Autodesk Inventor part; units mm, degrees
ref_plane "YZ Plane" through (0, 0, 0) normal (1, 0, 0) x (0, 1, 0)
ref_plane "XZ Plane" through (0, 0, 0) normal (0, 1, 0) x (-1, 0, 0)
ref_plane "XY Plane" through (0, 0, 0) normal (0, 0, 1) x (1, 0, 0)
sketch "Sketch1" plane through (0, 0, 0) normal (0, 0, 1) x (1, 0, 0)
  line L0 (-30, 0) -> (0, 0)
  line L1 (100, 0) -> (0, 0)
  line L2 (100, 0) -> (100, -35)
  line L3 (100, -35) -> (5, -35)
  arc A0 (-30, 0) -> (5, -35) centre (5, 0) ccw
  dimension "d0" = 30
  dimension "d26" = 130
  dimension "d27" = 35
  dimension "d28" = 35
extrude "Extrusion1" add sketch "Sketch1" against normal blind 50
sketch "Sketch2" plane through (-30, 0, 0) normal (0, 1, 0) x (1, 0, 0)
  circle A0 centre (110, 25) radius 12.5
  circle A1 centre (110, 25) radius 35
  line L0 (0, 0) -> (0, 50)
  line L1 (0, 25) -> (130, 25)
  line L2 (130, 0) -> (130, 50)
  point P0 (30, 0)
  dimension "d6" = 25
  dimension "d7" = 70
  dimension "d8" = 110
extrude "Extrusion4" add sketch "Sketch2" against normal up to surface (35 mm away) contours L1 A0 | A1 | A0 L1
sketch "Sketch4" plane through (-30, 0, 0) normal (0, 1, 0) x (1, 0, 0)
  line L0 (85.5051, 0) -> (0, 0)
  line L1 (19, 0) -> (19, 9)
  line L2 (19, 9) -> (12, 9)
  line L3 (12, 9) -> (12, 12)
  line L4 (12, 12) -> (19, 12)
  line L5 (19, 12) -> (19, 27)
  line L6 (19, 27) -> (9, 27)
  line L7 (9, 27) -> (9, 47)
  line L8 (9, 47) -> (76, 47)
  line L9 (76, 47) -> (76, 0)
  line L10 (71, 0) -> (71, 42)
  line L11 (71, 42) -> (19, 42)
  line L12 (19, 42) -> (19, 40)
  line L13 (19, 40) -> (59, 40)
  line L14 (59, 40) -> (59, 12)
  line L15 (59, 12) -> (66, 12)
  line L16 (66, 12) -> (66, 9)
  line L17 (66, 9) -> (59, 9)
  line L18 (59, 9) -> (59, 0)
  point P0 (30, 0)
  point P1 (12, 10.5)
  point P2 (66, 10.5)
  dimension "d31" = 54
  dimension "d32" = 36
  dimension "d33" = 7
  dimension "d34" = 7
  dimension "d35" = 40
  dimension "d36" = 2
  dimension "d37" = 3
  dimension "d38" = 9
  dimension "d39" = 15
  dimension "d40" = 10
  dimension "d41" = 20
  dimension "d42" = 5
  dimension "d43" = 67
extrude "Extrusion5" cut sketch "Sketch4" against normal blind 10 contours L0 L10 L11 L12 L13 L14 L15 L16 L17 L18 L1 L2 L3 L4 L5 L6 L7 L8 L9
sketch "Sketch5" plane through (-30, 0, 0) normal (0, 1, 0) x (1, 0, 0)
  arc A0 (85.5051, 0) -> (85.5051, 50) centre (110, 25) ccw
  circle A1 centre (110, 25) radius 35
  circle A2 centre (110, 25) radius 12.5
  point P0 (30, 0)
  point P1 (85.5051, 50)
  point P2 (85.5051, 0)
  dimension "d46" = 25
extrude "Extrusion6" cut sketch "Sketch5" against normal blind 22.5 contours A1 A0 | A2
sketch "Sketch6" plane through (-30, -22.5, 0) normal (0, 1, 0) x (1, 0, 0)
  arc A0 (85.5051, 0) -> (85.5051, 50) centre (110, 25) ccw
  arc A1 (85.5051, 50) -> (85.5051, 0) centre (110, 25) ccw
  circle A2 centre (110, 25) radius 12.5
  point P0 (30, 0)
  dimension "d49" = 25
extrude "Extrusion7" cut sketch "Sketch6" against normal blind 5 contours A2
properties part number "wirst 2 left"
Part model, mm, in its own coordinate system. A direction names the side the tool comes from. Give positions to 0.01 mm unless a question says otherwise; leave off trailing zeros. Order: outer loops, then holes, each group sorted by start corner. A loop starts at its lowest first (then second) coordinate and runs counter-clockwise, first axis right, second up. Notation, with made-up numbers: (-23, 39.5) - (21, 39.5) arc R9 cw to (21, 56.5) - close; hole circle Ø7 at (41.25, 72.5). An arc over 180 degrees is marked (long way). Use a Markdown table: item, result.
1) Flat gauge pins, fed straight in: P1, Ø8, axis at x = 72.5, z = -2, coming from the +Y side; P2, Ø8, axis at y = -11.5, z = -8, coming from the +X side; P3, Ø5, axis at y = -6.5, z = -15, coming from the +X side. Where does each tip first touch, or does it go through?
Checked values:
| item | result |
|---|---|
| P1 | y = -22.5 |
| P2 | x = 52 |
| P3 | x = 47.31 |
2) Saw through at C-C on y = -3. List the corners of the cut face in (x, z).
Checked values:
| item | result |
|---|---|
| outline | (-29.87, -50) - (55.51, -50) arc R35 cw to (46, -33.31) - (46, -47) - (-21, -47) - (-21, -27) - (-11, -27) - (-11, -12) - (-18, -12) - (-18, -9) - (-11, -9) - (-11, 0) - (-29.87, 0) - close; (-11, -42) - (41, -42) - (41, 0) - (29, 0) - (29, -9) - (36, -9) - (36, -12) - (29, -12) - (29, -40) - (-11, -40) - close; (46, -16.69) arc R35 cw to (55.51, 0) - (46, 0) - close |
3) Saw through at A-A on x = 80. List the corners of the cut face in (y, z).
Checked values:
| item | result |
|---|---|
| outline | (-35, -60) - (-22.5, -60) - (-22.5, -37.5) - (-27.5, -37.5) - (-27.5, -12.5) - (-22.5, -12.5) - (-22.5, 10) - (-35, 10) - close |
4) 3-axis set-ups, long thin cutter, end or side, ignore diameter. For faces 1 (the flat face through (29, -5, -5)), 2 (the flat face through (36, -5, -11)), 3 (the cylindrical face through (-20.019, -24.475, -24.65)): which of +Z, -Z, +X, -X, +Y, -Y reach the whole face in a straight line?
Checked values:
| item | result |
|---|---|
| face 1 | +Z, +Y |
| face 2 | +Y |
| face 3 | +Z, -Z, -X, -Y |
5) Two-plate mould, pull along X, no slides. Class faces 4 (the flat face through (-15, -5, -12)), 5 (the flat face through (32, -5, -12)), 6 (the cylindrical face through (45, -11, -25)), 7 (the flat face through (49, 0, -5)): +X half, -X half, draft (parallel to the pull), parting line (faces both ways), or undercut.
Checked values:
| item | result |
|---|---|
| face 4 | undercut |
| face 5 | undercut |
| face 6 | +X half |
| face 7 | draft |
6) Probe L1, parallel to Z at x = -16, y = -3; L2, parallel to Z at x = 80, y = -25.05; L3, parallel to X at y = -7.5, z = -11. List the from-to ranges inside material, lowest first. Write a range as from..to.
Checked values:
| item | result |
|---|---|
| L1 | -50..-47, -27..-12, -9..0 |
| L2 | -60..-37.5, -12.5..10 |
| L3 | -29.19..-18, 36..41, 46..47.92 |
7) Saw through at B-B on z = -25. List the corners of the cut face in (x, y).
Checked values:
| item | result |
|---|---|
| outline | (-30, 0) arc R35 ccw to (5, -35) - (115, -35) - (115, -22.5) - (92.5, -22.5) - (92.5, -27.5) - (67.5, -27.5) - (67.5, -22.5) - (45, -22.5) - (45, -10) - (41, -10) - (41, 0) - (29, 0) - (29, -10) - (-11, -10) - (-11, 0) - close |
8) Saw through at D-D on x = -13. List the corners of the cut face in (y, z), plus the area to 3 significant figures.
Checked values:
| item | result |
|---|---|
| outline | (-30.02, -50) - (0, -50) - (0, -47) - (-10, -47) - (-10, -27) - (0, -27) - (0, -12) - (-10, -12) - (-10, -9) - (0, -9) - (0, 0) - (-30.02, 0) - close |
| area | 1,270 mm² |
